Read the model definition and answer for the solid it produces. Units are mm, in the model's axes. Coordinates: 2 decimals unless noted, no trailing zeros. Loops run counter-clockwise (first coordinate to the right, second up) from the corner with the lowest first, then second, coordinate; pieces in that order, holes last. Notation, with made-up numbers: (35.25, -33) - (89.25, -33) arc R12 ccw to (89.25, -12) - close; hole circle Ø4 at (-31.5, 85). An arc over 180 degrees is marked (long way). Use CSV: the item, a comma, the result in double quotes.
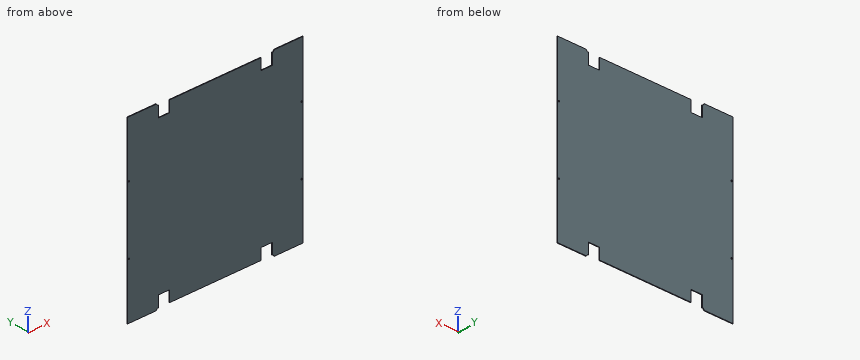
```python
from build123d import *

# Parameters (mm, degrees)
BOSS_EXTRUDE1_DEPTH          = 1.5875
F_1_8_0_125_DIAMETER_HOLE1_D = 3.175


with BuildPart() as part:
    # Sketch1 → Boss-Extrude1 (new body)
    with BuildSketch(Plane(origin=(0, 0, 0), x_dir=(1, 0, 0), z_dir=(0, 1, 0))):
        with BuildLine():
            ThreePointArc((-132.542154043, 202.449520044), (-135.236230879, 203.565443208), (-136.352154043, 206.259520044))
            Line((-136.352154043, 206.259520044), (-202.392154043, 206.259520044))
            Line((-202.392154043, 206.259520044), (-202.392154043, -200.140479956))
            Line((-202.392154043, -200.140479956), (-136.352154043, -200.140479956))
            ThreePointArc((-136.352154043, -200.140479956), (-135.236230879, -197.44640312), (-132.542154043, -196.330479956))
            Line((-132.542154043, -196.330479956), (-132.542154043, -170.930479956))
            Line((-132.542154043, -170.930479956), (-107.142154043, -170.930479956))
            Line((-107.142154043, -170.930479956), (-107.142154043, -196.330479956))
            Line((-107.142154043, -196.330479956), (101.137845957, -196.330479956))
            Line((101.137845957, -196.330479956), (101.137845957, -170.930479956))
            Line((101.137845957, -170.930479956), (126.537845957, -170.930479956))
            Line((126.537845957, -170.930479956), (126.537845957, -196.330479956))
            ThreePointArc((126.537845957, -196.330479956), (129.231922793, -197.44640312), (130.347845957, -200.140479956))
            Line((130.347845957, -200.140479956), (196.387845957, -200.140479956))
            Line((196.387845957, -200.140479956), (196.387845957, 206.259520044))
            Line((196.387845957, 206.259520044), (130.347845957, 206.259520044))
            ThreePointArc((130.347845957, 206.259520044), (129.231922793, 203.565443208), (126.537845957, 202.449520044))
            Line((126.537845957, 202.449520044), (126.537845957, 177.049520044))
            Line((126.537845957, 177.049520044), (101.137845957, 177.049520044))
            Line((101.137845957, 177.049520044), (101.137845957, 202.449520044))
            Line((101.137845957, 202.449520044), (-107.142154043, 202.449520044))
            Line((-107.142154043, 202.449520044), (-107.142154043, 177.049520044))
            Line((-107.142154043, 177.049520044), (-132.542154043, 177.049520044))
            Line((-132.542154043, 177.049520044), (-132.542154043, 202.449520044))
        make_face()
    extrude(amount=BOSS_EXTRUDE1_DEPTH)

    # 1/8 (0.125) Diameter Hole1 (through all)
    with Locations(Plane(origin=(0, 1.5875, 0), x_dir=(1, 0, 0), z_dir=(0, 1, 0))):
        with Locations((-199.217154043, 79.259520044), (-199.217154043, -73.140479956), (193.212845957, -73.140479956), (193.212845957, 79.259520044)):
            Hole(F_1_8_0_125_DIAMETER_HOLE1_D / 2)


solid = part.part
```
Q1. The part is cut by section B-B on x = 81. Determine the outline of the cut face in (y, z).
Reported:
outline,"(0, -202.45) - (1.59, -202.45) - (1.59, 196.33) - (0, 196.33) - close"
Q2. Find the intervals of material crossed by probe 1 along Z at (x, y) = (64.5, 0.4); probe 2 along Z at (x, y) = (-117, 0.35), in increasing order. Write a range as [from, to].
Reported:
probe 1,"z = [-202.45, 196.33]"
probe 2,"z = [-177.05, 170.93]"
Q3. The part is cut by section A-A on y = 0.55. Determine the outline of the cut face in (x, z) (1 decimal).
Reported:
outline,"(-202.4, -206.3) - (-136.4, -206.3) arc R3.8 cw to (-132.5, -202.4) - (-132.5, -177) - (-107.1, -177) - (-107.1, -202.4) - (101.1, -202.4) - (101.1, -177) - (126.5, -177) - (126.5, -202.4) arc R3.8 cw to (130.3, -206.3) - (196.4, -206.3) - (196.4, 200.1) - (130.3, 200.1) arc R3.8 cw to (126.5, 196.3) - (126.5, 170.9) - (101.1, 170.9) - (101.1, 196.3) - (-107.1, 196.3) - (-107.1, 170.9) - (-132.5, 170.9) - (-132.5, 196.3) arc R3.8 cw to (-136.4, 200.1) - (-202.4, 200.1) - close; hole circle Ø3.2 at (-199.2, -79.3); hole circle Ø3.2 at (-199.2, 73.1); hole circle Ø3.2 at (193.2, -79.3); hole circle Ø3.2 at (193.2, 73.1)"
Q4. Given P1, Ø0.8, axis at x = -114.5, y = 0.5, coming from the -Z side; P2, Ø1.9, axis at x = 193.21, z = 73.14, coming from the -Y side; P3, Ø5, axis at x = 193.21, z = -79.26, coming from the +Y side; P4, Ø0.5, axis at x = 116.5, y = 1, coming from the +Z side, each flat-ended and moving along its own axis, determine where each tip first touches the part or whether it passes through.
Reported:
P1,"stops at z = -177.05"
P2,"passes through"
P3,"stops at y = 1.59"
P4,"stops at z = 170.93"
